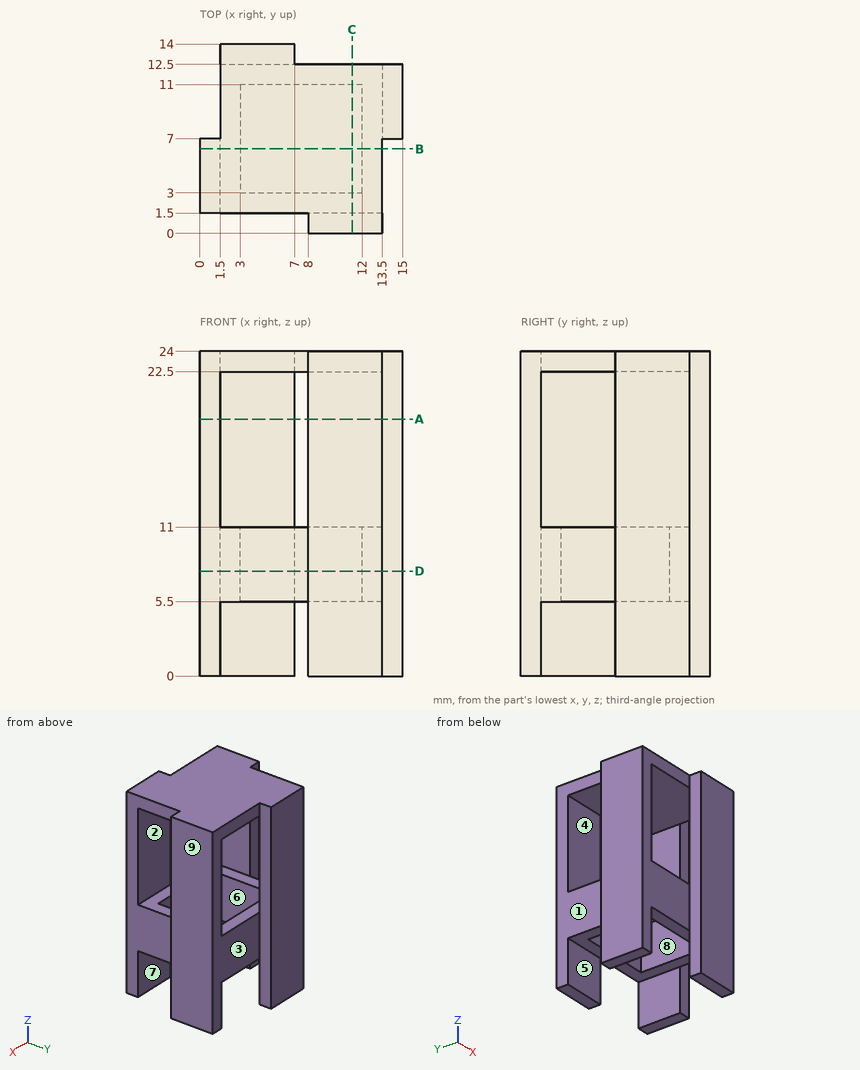
Geometry: see drawing. Coordinates: mm, zero at the bounding-box minimum. A direction names the side the tool comes from. Give positions to 0.01 mm unless a question says otherwise; leave off trailing zeros. Order: outer loops, then holes, each group sorted by start corner. A loop starts at its lowest first (then second) coordinate and runs counter-clockwise, first axis right, second up.
1. Cut plane D-D (z = 7.75). Return loops of the section in (x, y), and give its area (3 significant figures).
Computed:
outline: (0, 1.5) - (8, 1.5) - (8, 0) - (13.5, 0) - (13.5, 7) - (15, 7) - (15, 12.5) - (7, 12.5) - (7, 14) - (1.5, 14) - (1.5, 7) - (0, 7) - close; hole (3, 3) - (12, 3) - (12, 11) - (3, 11) - close
area: 93.0 mm2
2. Draft query along X for the marked faces 6, 7, 8 and 9. Return one class per face: released by +X, released by -X, zero draft, split by the parting line, or undercut.
Computed:
face 6: undercut
face 7: zero draft
face 8: undercut
face 9: released by +X
3. Cut plane A-A (z = 19). Return loops of the section in (x, y).
Computed:
outline: (0, 1.5) - (1.5, 1.5) - (1.5, 7) - (0, 7) - close; (1.5, 12.5) - (7, 12.5) - (7, 14) - (1.5, 14) - close; (8, 0) - (13.5, 0) - (13.5, 1.5) - (8, 1.5) - close; (13.5, 7) - (15, 7) - (15, 12.5) - (13.5, 12.5) - close
4. Cut plane B-B (y = 6.25). Return loops of the section in (x, z).
Computed:
outline: (0, 0) - (1.5, 0) - (1.5, 5.5) - (3, 5.5) - (3, 11) - (1.5, 11) - (1.5, 22.5) - (13.5, 22.5) - (13.5, 24) - (0, 24) - close; (12, 5.5) - (13.5, 5.5) - (13.5, 11) - (12, 11) - close
5. Cut plane C-C (x = 11.25). Return loops of the section in (y, z).
Computed:
outline: (0, 0) - (1.5, 0) - (1.5, 5.5) - (3, 5.5) - (3, 11) - (1.5, 11) - (1.5, 22.5) - (12.5, 22.5) - (12.5, 24) - (0, 24) - close; (11, 5.5) - (12.5, 5.5) - (12.5, 11) - (11, 11) - close
6. Line query: probe 1 along X at (y, z) = (10.5, 8.25); probe 2 along Z at (x, y) = (12.25, 2); probe 3 along Y at (x, z) = (3.5, 7). Output: solid intervals per line, ascending.
Computed:
probe 1: x = 1.5 to 3, 12 to 15
probe 2: z = 5.5 to 11, 22.5 to 24
probe 3: y = 1.5 to 3, 11 to 14
7. Set-up query: the marked faces 1, 2, 3, 4 and 5. Return all of +Z, -Z, +X, -X, +Y, -Y with unobstructed straight access to the full face (end or side cutting, diameter ignored); none if empty.
Computed:
face 1: +Z, -Z, -X, +Y
face 2: +X, +Y
face 3: +Z, -Z, +X, +Y
face 4: -X, -Y
face 5: -Z, -X, -Y
8. Pin query (flat end, axial travel): pin 1 Ø3 at (y, z) = (10, 2) entering from -X; pin 2 Ø2.5 at (x, z) = (11.5, 13.5) entering from +Y; pin 3 Ø1.6 at (y, z) = (3, 19.5) entering from +X; pin 4 Ø3 at (x, z) = (8.5, 9.5) entering from -Y. Return the tip coordinate at first contact, or that it passes through.
Computed:
pin 1: stops at x = 13.5
pin 2: stops at y = 1.5
pin 3: stops at x = 1.5
pin 4: stops at y = 0
